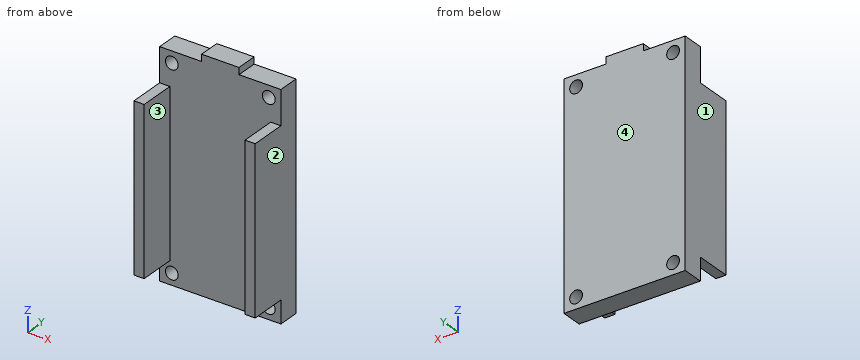
from build123d import *

# Parameters (mm, degrees)
SKETCH1_W           = 28.5
SKETCH1_H           = 51.8
SKETCH1_R           = 1.5
SKETCH1_W_2         = 8.8
SKETCH1_H_2         = 1.6
BOSS_EXTRUDE1_DEPTH = 5
SKETCH2_W           = 2.4
SKETCH2_H           = 38.5
BOSS_EXTRUDE2_DEPTH = 8.5


with BuildPart() as part:
    # Sketch1 → Boss-Extrude1 (new body)
    # profile 1 of 2: a face of its own
    with BuildSketch(Plane(origin=(0, 0, 0), x_dir=(1, 0, 0), z_dir=(0, 1, 0))):
        Rectangle(SKETCH1_W, SKETCH1_H)
        with Locations(Location((-11.4, -23.2, 0), (0, 0, 270))):
            Circle(SKETCH1_R, mode=Mode.SUBTRACT)
        with Locations(Location((11.4, -23.2, 0), (0, 0, 270))):
            Circle(SKETCH1_R, mode=Mode.SUBTRACT)
        with Locations(Location((11.4, 23.2, 0), (0, 0, 270))):
            Circle(SKETCH1_R, mode=Mode.SUBTRACT)
        with Locations(Location((-11.4, 23.2, 0), (0, 0, 270))):
            Circle(SKETCH1_R, mode=Mode.SUBTRACT)
    # profile 2 of 2: a face of its own
    with BuildSketch(Plane(origin=(0, 0, 0), x_dir=(1, 0, 0), z_dir=(0, 1, 0))):
        with Locations((0, -26.7)):
            Rectangle(SKETCH1_W_2, SKETCH1_H_2)
    extrude(amount=BOSS_EXTRUDE1_DEPTH)

    # Sketch2 → Boss-Extrude2 (add)
    with BuildSketch(Plane.XZ):
        with Locations((13.05, -1.35)):
            Rectangle(SKETCH2_W, SKETCH2_H)
        with Locations((-13.05, -1.35)):
            Rectangle(SKETCH2_W, SKETCH2_H)
    extrude(amount=BOSS_EXTRUDE2_DEPTH)


solid = part.part
Geometry check sheet. Reference: the model listing, model coordinates, mm. Face numbers are marked on the shaded views. Round coordinates to 2 decimals unless told otherwise and drop trailing zeros. Loops run counter-clockwise (first coordinate to the right, second up) from the corner with the lowest first, then second, coordinate; pieces in that order, holes last.
Item 1: Gauge pin test, flat ends, axial feed: pin 1 (1.8 mm diameter, centred on x = -11.4, z = 23.2, fed in from -Y); pin 2 (6 mm diameter, centred on x = -7, z = 16.5, fed in from -Y); pin 3 (5.5 mm diameter, centred on x = -8, y = 3.5, fed in from +Z); pin 4 (1.9 mm diameter, centred on x = -12.5, y = -4, fed in from -Z). Record the tip position at first contact, or that the pin passes through.
Item 2: Cross-section at A-A on z = -23.2. Record the boundary of the cut face in (x, y).
Item 3: Cross-section at C-C on z = -1.5. Record the boundary of the cut face in (x, y), then the cut area to 3 significant figures.
Item 4: Cross-section at B-B on y = -7. Record the boundary of the cut face in (x, z).
Item 5: Mould release check, pull along X, two halves, no side actions. Record for the marked faces 1, 2, 3 and 4: pulls with the +X half, pulls with the -X half, needs draft (parallel to the pull), parting line crosses it, or undercut.
Item 6: Cross-section at D-D on x = 7.5. Record the boundary of the cut face in (y, z), then the cut area to 3 significant figures.
Item 7: Thickness scan on line 1 (X direction, y = 2, z = 23.2); line 2 (X direction, y = -5.5, z = -13.5); line 3 (Y direction, x = 4.25, z = -10). Record the ranges inside material, lowest first.
Answer sheet:
1. pin 1: passes through
1. pin 2: stops at y = 0
1. pin 3: stops at z = 25.9
1. pin 4: stops at z = -20.6
2. outline: (-14.25, 0) - (-12.9, 0) - (-12.9, 5) - (-14.25, 5) - close; (-9.9, 0) - (9.9, 0) - (9.9, 5) - (-9.9, 5) - close; (12.9, 0) - (14.25, 0) - (14.25, 5) - (12.9, 5) - close
3. outline: (-14.25, -8.5) - (-11.85, -8.5) - (-11.85, 0) - (11.85, 0) - (11.85, -8.5) - (14.25, -8.5) - (14.25, 5) - (-14.25, 5) - close
3. area: 183 mm2
4. outline: (-14.25, -20.6) - (-11.85, -20.6) - (-11.85, 17.9) - (-14.25, 17.9) - close; (11.85, -20.6) - (14.25, -20.6) - (14.25, 17.9) - (11.85, 17.9) - close
5. face 1: pulls with the -X half
5. face 2: pulls with the +X half
5. face 3: undercut
5. face 4: needs draft
6. outline: (0, -25.9) - (5, -25.9) - (5, 25.9) - (0, 25.9) - close
6. area: 259 mm2
7. line 1: x = -14.25 to -12.9, -9.9 to 9.9, 12.9 to 14.25
7. line 2: x = -14.25 to -11.85, 11.85 to 14.25
7. line 3: y = 0 to 5
